Autodesk Inventor part; units mm, degrees
ref_plane "YZ Plane" through (0, 0, 0) normal (1, 0, 0) x (0, 1, 0)
ref_plane "XZ Plane" through (0, 0, 0) normal (0, 1, 0) x (-1, 0, 0)
ref_plane "XY Plane" through (0, 0, 0) normal (0, 0, 1) x (1, 0, 0)
sketch "Sketch1" plane through (0, 0, 0) normal (0, 0, 1) x (1, 0, 0)
  line L0 (-79.121, 7.62) -> (-79.121, -7.62)
  line L1 (-79.121, -7.62) -> (-84.201, -7.62)
  line L2 (-84.201, 7.62) -> (-79.121, 7.62)
  line L3 (-80.391, -7.62) -> (-92.71, -7.62)
  line L4 (-92.71, -7.62) -> (-92.71, 7.62) construction
  line L5 (-92.71, 7.62) -> (-80.391, 7.62)
  line L6 (-80.391, 7.62) -> (-80.391, -7.62)
  arc A0 (-92.71, 7.62) -> (-92.71, -7.62) centre (-92.71, 0) ccw
  arc A1 (-92.71, -7.62) -> (-92.71, 7.62) centre (-92.71, 0) ccw construction
  line L7 (-92.71, 0) -> (-100.33, 0) construction
  point P0 (0, 0)
  dimension "d0" = 1.27
  dimension "d1" = 19.939
extrude "Extrusion1" add sketch "Sketch1" along normal mid plane 48.26 contours L6 L1 L3 A0 L5 L2
sketch "Sketch2" plane through (-92.71, 7.62, 24.13) normal (0, 1, 0) x (1, 0, 0)
  circle A0 centre (8.509, 11.43) radius 1.5875
  circle A1 centre (8.509, 36.83) radius 1.5875
  circle A2 centre (8.509, 11.43) radius 1.5875
  circle A3 centre (8.509, 36.83) radius 1.5875
  point P0 (92.71, 24.13)
extrude "Extrusion2" cut sketch "Sketch2" against normal through all
sketch "Sketch3" plane through (-92.71, 7.62, 24.13) normal (0, 1, 0) x (1, 0, 0)
  line L0 (0, 48.26) -> (-7.62, 48.26)
  line L1 (0, 48.26) -> (12.319, 48.26)
  line L2 (-7.62, 0) -> (0, 0)
  line L3 (12.319, 0) -> (0, 0)
  circle A0 centre (8.509, 11.43) radius 1.5875
  circle A1 centre (8.509, 36.83) radius 1.5875
  line L4 (12.319, 48.26) -> (12.319, 0)
  arc A2 (7.62, 15.1348) -> (7.62, 7.7252) centre (8.509, 11.43) ccw
  circle A3 centre (8.509, 36.83) radius 1.5875
  arc A4 (7.62, 40.5348) -> (7.62, 33.1252) centre (8.509, 36.83) ccw
  line L5 (-7.62, 48.26) -> (-7.62, 0)
  line L6 (-7.62, 24.13) -> (12.319, 24.13) construction
  line L7 (-7.62, 41.91) -> (7.62, 41.91)
  line L8 (7.62, 41.91) -> (7.62, 40.5348)
  line L9 (7.62, 6.35) -> (-7.62, 6.35)
  line L10 (-7.62, 6.35) -> (-7.62, 41.91)
  line L11 (-7.62, 41.91) -> (7.62, 6.35) construction
  line L12 (7.62, 41.91) -> (-7.62, 6.35) construction
  line L13 (7.62, 40.5348) -> (7.62, 33.1252) construction
  arc A5 (12.319, 36.83) -> (7.62, 40.5348) centre (8.509, 36.83) ccw construction
  arc A6 (7.62, 33.1252) -> (12.319, 36.83) centre (8.509, 36.83) ccw construction
  line L14 (7.62, 33.1252) -> (7.62, 15.1348)
  line L15 (7.62, 15.1348) -> (7.62, 7.7252) construction
  arc A7 (12.319, 11.43) -> (7.62, 15.1348) centre (8.509, 11.43) ccw construction
  arc A8 (7.62, 7.7252) -> (12.319, 11.43) centre (8.509, 11.43) ccw construction
  line L16 (7.62, 7.7252) -> (7.62, 6.35)
  point P0 (92.71, 24.13)
  point P1 (0, 24.13)
  dimension "d17" = 35.56
  dimension "d18" = 15.24
extrude "Extrusion3" cut sketch "Sketch3" against normal through all contours L7 L8 A4 L14 A2 L16 L9 L5
sketch "Sketch4" plane through (0, 0, 0) normal (0, 0, 1) x (1, 0, 0)
  arc A0 (-92.71, 7.62) -> (-92.71, -7.62) centre (-92.71, 0) ccw
  circle A1 centre (-92.71, 0) radius 2.54
  point P0 (0, 0)
  dimension "d11" = 5.08
extrude "Extrusion4" cut sketch "Sketch4" along normal mid plane 43.18
sketch "Sketch5" plane through (0, 0, 24.13) normal (0, 0, 1) x (1, 0, 0)
  line L0 (-80.391, -7.62) -> (-80.391, 7.62)
  line L1 (-80.391, 7.62) -> (-92.71, 7.62)
  arc A0 (-92.71, 7.62) -> (-92.71, -7.62) centre (-92.71, 0) ccw
  line L2 (-92.71, -7.62) -> (-80.391, -7.62)
  arc A1 (-92.71, 6.35) -> (-92.71, -6.35) centre (-92.71, 0) ccw
  line L3 (-92.71, 6.35) -> (-81.661, 6.35)
  line L4 (-81.661, 6.35) -> (-81.661, -6.35) construction
  line L5 (-81.661, -6.35) -> (-92.71, -6.35)
  line L6 (-81.661, 6.35) -> (-80.391, 6.35)
  line L7 (-81.661, -6.35) -> (-80.391, -6.35)
  line L8 (-80.391, 7.62) -> (-80.391, -7.62)
  point P0 (0, 0)
  dimension "d14" = 1.27
extrude "Extrusion5" cut sketch "Sketch5" against normal blind 3.81 contours L7 L5 A1 L3 L6 L0
mirror "Mirror1" about plane through (0, 0, 0) normal (0, 0, 1) of "Extrusion5"
properties part number "Steering_Arm"
Geometry: final body of the model. Coordinates: model frame, mm. A direction names the side the tool comes from. Round coordinates to 2 decimals unless told otherwise and drop trailing zeros. Loops run counter-clockwise (first coordinate to the right, second up) from the corner with the lowest first, then second, coordinate; pieces in that order, holes last. Notation, with made-up numbers: M 68.5,58.5 L 73.5,58.5 A25 cw 73.5,95.5 Z; hole C 69,25 d11. An arc over 180 degrees is marked long. One line per question, with ' | ' between items.
(1) Cut plane A-A on y = 0. Give the number of separate pieces and of enclosed holes in the cut face, plus the area to 3 significant figures.
Check result:
separate pieces: 3 | enclosed holes: 2 | area: 269 mm2
(2) Access query for faces 1 (the flat face through (-87, 6.35, 22)), 2 (the flat face through (-86, -6.35, -22)), 3 (the flat face through (-85.09, 0, 17)). Directions: +Z, -Z, +X, -X, +Y, -Y. A direction counts if a zero-diameter tool reaches every point of the face in a straight line with its end or side. Return the directions, or none.
Check result:
face 1: +Z, +X | face 2: -Z, +X | face 3: -X, +Y, -Y
(3) Cut plane B-B on x = -81.75. Return the cut outline in (y, z), plus the area to 3 significant figures.
Check result:
outline: M -7.62,-24.13 L -6.35,-24.13 L -6.35,-20.32 L 6.35,-20.32 L 6.35,-24.13 L 7.62,-24.13 L 7.62,24.13 L 6.35,24.13 L 6.35,20.32 L -6.35,20.32 L -6.35,24.13 L -7.62,24.13 Z | area: 639 mm2
(4) Cut plane D-D on z = -18.5. Return the cut outline in (x, y), plus the area to 3 significant figures.
Check result:
outline: M -92.71,-7.62 L -80.39,-7.62 L -80.39,7.62 L -92.71,7.62 A7.62 ccw Z; hole C -92.71,0 d5.08 | area: 259 mm2
(5) Cut plane C-C on z = 12.7. Return the cut outline in (x, y), plus the area to 3 significant figures.
Check result:
outline: M -88.01,-7.62 L -85.79,-7.62 L -85.79,7.62 L -88.01,7.62 Z; M -82.61,-7.62 L -80.39,-7.62 L -80.39,7.62 L -82.61,7.62 Z | area: 67.7 mm2
(6) Pull-direction query (Z, two-part tool) for faces 4 (the cylindrical face through (-99.06, -0.14, -22.25)), 5 (the flat face through (-90, 0, -20.32)), 6 (the flat face through (-92, -7, 24.13)), 7 (the flat face through (-89, 0, 17.78)); classes: +Z half, -Z half, draft (parallel to the pull), parting line (faces both ways), or undercut.
Check result:
face 4: draft | face 5: -Z half | face 6: +Z half | face 7: undercut
(7) Material intervals for line 1 along Z through (x, y) = (-94.5, 4); line 2 along Z through (x, y) = (-85.5, 2); line 3 along Y through (x, z) = (-92.71, -19.15), sorted ascending. Write a range as from..to.
Check result:
line 1: z = -20.32..-17.78, 17.78..20.32 | line 2: z = -20.32..-17.78, -16.28..-13.61, -11.79..-9.12, 9.12..11.79, 13.61..16.28, 17.78..20.32 | line 3: y = -7.62..-2.54, 2.54..7.62
(8) Contact query for flat-ended pins moving along their axis: P1, Ø7.5, axis at x = -92, y = 3.5, coming from the -Z side; P2, Ø1, axis at x = -95, y = 2.5, coming from the +Z side; P3, Ø1.5, axis at y = 3, z = 17.5, coming from the -X side; P4, Ø4, axis at x = -95, z = -19, coming from the +Y side. Output: stop coordinate, or through.
Check result:
P1: stops at z = -24.13 | P2: stops at z = 20.32 | P3: stops at x = -99.97 | P4: stops at y = 7.61
